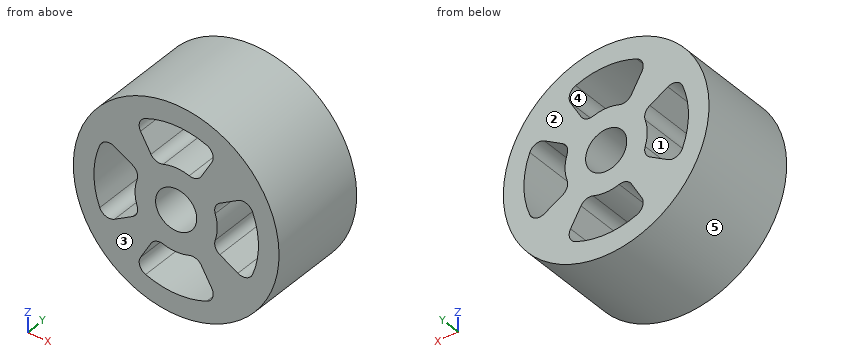
from build123d import *

# Parameters (mm, degrees)
SKETCH_1_R      = 20
SKETCH_1_R_2    = 4
EXTRUDE_1_DEPTH = 20
FILLET_1_R      = 2


with BuildPart() as part:
    # 草图1 → 凸台-拉伸1 (new body)
    with BuildSketch(Plane(origin=(0, 0, 0), x_dir=(1, 0, 0), z_dir=(0, 1, 0))):
        with Locations(Location((0, 0, 0), (0, 0, 270))):
            Circle(SKETCH_1_R)
        with Locations(Location((0, 0, 0), (0, 0, 270))):
            Circle(SKETCH_1_R_2, mode=Mode.SUBTRACT)
        with BuildLine():
            Line((-4, -6.92820323), (-8, -13.856406461))
            ThreePointArc((-8, -13.856406461), (0, -16), (8, -13.856406461))
            Line((8, -13.856406461), (4, -6.92820323))
            ThreePointArc((4, -6.92820323), (0, -8), (-4, -6.92820323))
        make_face(mode=Mode.SUBTRACT)
        with BuildLine():
            Line((-4, 6.92820323), (-8, 13.856406461))
            ThreePointArc((-8, 13.856406461), (0, 16), (8, 13.856406461))
            Line((8, 13.856406461), (4, 6.92820323))
            ThreePointArc((4, 6.92820323), (0, 8), (-4, 6.92820323))
        make_face(mode=Mode.SUBTRACT)
        with BuildLine():
            Line((-6.92820323, 4), (-13.856406461, 8))
            ThreePointArc((-13.856406461, 8), (-16, 0), (-13.856406461, -8))
            Line((-13.856406461, -8), (-6.92820323, -4))
            ThreePointArc((-6.92820323, -4), (-8, 0), (-6.92820323, 4))
        make_face(mode=Mode.SUBTRACT)
        with BuildLine():
            Line((6.92820323, -4), (13.856406461, -8))
            ThreePointArc((13.856406461, -8), (16, 0), (13.856406461, 8))
            Line((13.856406461, 8), (6.92820323, 4))
            ThreePointArc((6.92820323, 4), (8, 0), (6.92820323, -4))
        make_face(mode=Mode.SUBTRACT)
    extrude(amount=EXTRUDE_1_DEPTH)

    # 圆角1
    fillet_1_edges = [part.edges().sort_by_distance(p)[0] for p in [
        (8, 10, -13.856406461),
        (-8, 10, -13.856406461),
        (-4, 10, -6.92820323),
        (4, 10, -6.92820323),
        (13.856406461, 10, 8),
        (13.856406461, 10, -8),
        (6.92820323, 10, -4),
        (6.92820323, 10, 4),
        (-8, 10, 13.856406461),
        (8, 10, 13.856406461),
        (4, 10, 6.92820323),
        (-4, 10, 6.92820323),
        (-13.856406461, 10, -8),
        (-13.856406461, 10, 8),
        (-6.92820323, 10, 4),
        (-6.92820323, 10, -4),
    ]]
    fillet(fillet_1_edges, radius=FILLET_1_R)


solid = part.part
Could you check a few things on this model? Use its own coordinates, in mm. Face numbers are marked on the shaded views. A direction names the side the tool comes from. Coordinates: 2 decimals unless noted, no trailing zeros. Order: outer loops, then holes, each group sorted by start corner. A loop starts at its lowest first (then second) coordinate and runs counter-clockwise, first axis right, second up. Notation, with made-up numbers: (82, 5.5) -> (111, 5.5) arc R33 ccw to (111, 38.5) -> close; hole circle Ø2 at (77.5, -1). An arc over 180 degrees is marked (long way). One line per question, with ' | ' between items.
Q1. Imagine slicing it at B-B on x = 0. Please give me the cut outline in (y, z), and give its area (3 significant figures).
Return value:
outline: (0, -20) -> (20, -20) -> (20, -16) -> (0, -16) -> close; (0, -8) -> (20, -8) -> (20, -4) -> (0, -4) -> close; (0, 4) -> (20, 4) -> (20, 8) -> (0, 8) -> close; (0, 16) -> (20, 16) -> (20, 20) -> (0, 20) -> close | area: 320 mm²
Q2. Thinking about a two-plate mould opening in Z: for the marked faces 3, 4 and 5, which applies, pulls with the +Z half, pulls with the -Z half, needs draft (parallel to the pull), parting line crosses it, or undercut?
Return value:
face 3: needs draft | face 4: undercut | face 5: parting line crosses it
Q3. I'm going to push flat-ended pins straight in: P1, Ø5, axis at y = 6.5, z = 8.5, coming from the +X side; P2, Ø5, axis at y = 13, z = 1.5, coming from the -X side; P3, Ø3, axis at x = 14, y = 10.5, coming from the -Z side. Where does each tip first touch, or does it pass through?
Return value:
P1: x = 19.08 | P2: x = -20 | P3: z = -15.61
Q4. If I drill on L1, parallel to Z at x = 2, y = 5.5; L2, parallel to X at y = 3.75, z = 7 (3 decimals); L3, parallel to Z at x = -5, y = 10.25, over which ranges is the centre line in solid material (lowest first)?
Return value:
L1: -19.9 to -15.87, -7.75 to -3.46, 3.46 to 7.75, 15.87 to 19.9 | L2: -18.735 to -13.864, -12.136 to 12.136, 13.864 to 18.735 | L3: -19.36 to -15.2, -8.66 to 8.66, 15.2 to 19.36
Q5. Imagine slicing it at D-D on x = 10.5. Please give me the cut outline in (y, z).
Return value:
outline: (0, -17.02) -> (20, -17.02) -> (20, -6.06) -> (0, -6.06) -> close; (0, 6.06) -> (20, 6.06) -> (20, 17.02) -> (0, 17.02) -> close
Q6. Imagine slicing it at C-C on y = 10.25. State how many separate pieces and enclosed holes the cut face has, and give its area (3 significant figures).
Return value:
separate pieces: 1 | enclosed holes: 5 | area: 818 mm²
Q7. Imagine slicing it at A-A on z = 0. Please give me the cut outline in (x, y), and give its area (3 significant figures).
Return value:
outline: (-20, 0) -> (-16, 0) -> (-16, 20) -> (-20, 20) -> close; (-8, 0) -> (-4, 0) -> (-4, 20) -> (-8, 20) -> close; (4, 0) -> (8, 0) -> (8, 20) -> (4, 20) -> close; (16, 0) -> (20, 0) -> (20, 20) -> (16, 20) -> close | area: 320 mm²
Q8. On a 3-axis mill with a long thin cutter (end or side, diameter ignored), from which of +Z, -Z, +X, -X, +Y, -Y can I reach the whole of each face in a straight line? I mean the marked faces 1 and 2. Say none if no direction works.
Return value:
face 1: +Y, -Y | face 2: +Z, -Z, +X, -X, +Y
